Check sheet for the modelled part. Datum: model origin and axes. Units: mm. Face numbers are marked on the shaded views. A direction names the side the tool comes from. Coordinates: 2 decimals unless noted, no trailing zeros. Write each loop counter-clockwise with the first axis right and the second up, starting at its lowest first coordinate (ties: lowest second). Pieces come first, ordered by that corner, then holes. Notation, with made-up numbers: M -32,31.5 L -19,31.5 A13 ccw -19,38.5 Z; hole C 4.25,83.5 d4. An arc over 180 degrees is marked long. Answer as CSV lines item,"result". Start each with the question number.
Q1. Thickness scan on line 1 along X through (y, z) = (7.5, -7.5); line 2 along X through (y, z) = (20, 10.5); line 3 along Y through (x, z) = (-7.25, 10). Record the ranges inside material, lowest first. Write a range as from..to.
Q2. Sectioned sample at A-A, the plane y = 35. Record the cut outline in (x, z), then the cut area to 3 significant figures.
Q3. Access from +Z, -Z, +X, -X, +Y, -Y to the whole of each face (thin tool, end or side, straight path). Record for the marked faces 1, 2, 3 and 4.
Q4. Depth check by flat-ended pin: pin 1 Ø3 at (x, z) = (-5, -7.5) entering from -Y; pin 2 Ø10 at (x, z) = (0, 10) entering from -Y; pin 3 Ø3 at (x, y) = (-1.5, 7.5) entering from +Z; pin 4 Ø0.9 at (x, z) = (3.5, 11.5) entering from -Y. Enter the tip coordinate at first touch or a pass-through.
Q5. Sectioned sample at D-D, the plane x = 5. Record the cut outline in (y, z).
Q6. Sectioned sample at C-C, the plane z = -7.5. Record the cut outline in (x, y), then the cut area to 3 significant figures.
Q7. Sectioned sample at B-B, the plane x = -1.5. Record the cut outline in (y, z), then the cut area to 4 significant figures.
Q8. Mould release check, pull along X, two halves, no side actions. Record for the marked faces 5, 6, 7 and 8: pulls with the +X half, pulls with the -X half, needs draft (parallel to the pull), parting line crosses it, or undercut.
from build123d import *

# Parameters (mm, degrees)
BOSS_EXTRU_1_DEPTH      = 14
ESQUISSE2_W             = 20
ESQUISSE2_H             = 40
BOSS_EXTRU_2_DEPTH      = 15
ENL_V_MAT_EXTRU_1_REACH = 66.384
ENL_V_MAT_EXTRU_2_REACH = 49.418
ESQUISSE4_R             = 2


with BuildPart() as part:
    # Esquisse1 → Boss.-Extru.1 (new body)
    with BuildSketch(Plane(origin=(0, 0, 0), x_dir=(1, 0, 0), z_dir=(0, 1, 0))):
        Polygon((12.5, -12.5), (12.5, 0), (12.5, 12.5), (-12.5, 12.5), (-12.5, -12.5), align=None)
    extrude(amount=BOSS_EXTRU_1_DEPTH)

    # Esquisse2 → Boss.-Extru.2 (add)
    with BuildSketch(Plane.XY.offset(12.5)):
        Polygon((-12.5, 14), (12.5, 14), (12.5, 16.5), (12.5, 58), (-12.5, 58), align=None)
        with Locations((0, 36)):
            Rectangle(ESQUISSE2_W, ESQUISSE2_H, mode=Mode.SUBTRACT)
    extrude(amount=-BOSS_EXTRU_2_DEPTH)

    # Esquisse3 → Enlèv. mat.-Extru.1 (cut, up to next)
    with BuildSketch(Plane.ZY.offset(12.5), mode=Mode.PRIVATE) as enl_v_mat_extru_1_sk1:
        Polygon((12.5, 0), (4.5, 0), (4.5, 10), (9.5, 15), (12.5, 15), align=None)
    enl_v_mat_extru_1_tool1 = extrude(enl_v_mat_extru_1_sk1.sketch, amount=-ENL_V_MAT_EXTRU_1_REACH, mode=Mode.PRIVATE) & part.part
    add(enl_v_mat_extru_1_tool1.solids().sort_by_distance((-12.5, 6.821705, 8.771318))[0], mode=Mode.SUBTRACT)

    # Esquisse4 → Enlèv. mat.-Extru.2 (cut, up to next)
    with BuildSketch(Plane(origin=(0, 14, 0), x_dir=(1, 0, 0), z_dir=(0, 1, 0)), mode=Mode.PRIVATE) as enl_v_mat_extru_2_sk1:
        with Locations(Location((5, 7.5, 0), (0, 0, 270))):
            Circle(ESQUISSE4_R)
    enl_v_mat_extru_2_tool1 = extrude(enl_v_mat_extru_2_sk1.sketch, amount=-ENL_V_MAT_EXTRU_2_REACH, mode=Mode.PRIVATE) & part.part
    # Esquisse4 → Enlèv. mat.-Extru.2 (cut, up to next)
    with BuildSketch(Plane(origin=(0, 14, 0), x_dir=(1, 0, 0), z_dir=(0, 1, 0)), mode=Mode.PRIVATE) as enl_v_mat_extru_2_sk2:
        with Locations(Location((-5, 7.5, 0), (0, 0, 270))):
            Circle(ESQUISSE4_R)
    enl_v_mat_extru_2_tool2 = extrude(enl_v_mat_extru_2_sk2.sketch, amount=-ENL_V_MAT_EXTRU_2_REACH, mode=Mode.PRIVATE) & part.part
    add(enl_v_mat_extru_2_tool1.solids().sort_by_distance((5, 14, -7.5))[0], mode=Mode.SUBTRACT)
    add(enl_v_mat_extru_2_tool2.solids().sort_by_distance((-5, 14, -7.5))[0], mode=Mode.SUBTRACT)


solid = part.part
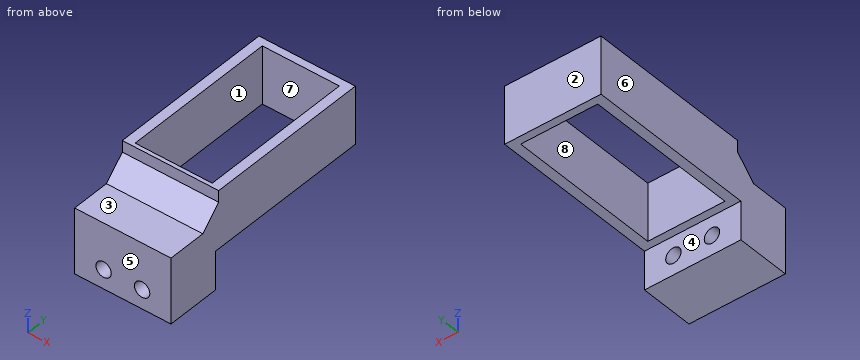
Output:
1,line 1,"x = -12.5..-7, -3..3, 7..12.5"
1,line 2,"x = -12.5..-10, 10..12.5"
1,line 3,"y = 15..16, 56..58"
2,outline,"M -12.5,-2.5 L -10,-2.5 L -10,12.5 L -12.5,12.5 Z; M 10,-2.5 L 12.5,-2.5 L 12.5,12.5 L 10,12.5 Z"
2,area,"75.0 mm^2"
3,face 1,"+Z, -Z"
3,face 2,"+Z, -Z, +X, -X, +Y"
3,face 3,"+Z, +X, -X, -Y"
3,face 4,"-Z, +X, -X, +Y"
4,pin 1,"passes through"
4,pin 2,"stops at y = 10.5"
4,pin 3,"stops at z = 4.5"
4,pin 4,"stops at y = 15"
5,outline,"M 0,-12.5 L 14,-12.5 L 14,-9.5 L 0,-9.5 Z; M 0,-5.5 L 14,-5.5 L 14,-2.5 L 16,-2.5 L 16,12.5 L 15,12.5 L 15,9.5 L 10,4.5 L 0,4.5 Z; M 56,-2.5 L 58,-2.5 L 58,12.5 L 56,12.5 Z"
6,outline,"M -12.5,0 L -7,0 L -7,14 L -12.5,14 Z; M -3,0 L 3,0 L 3,14 L -3,14 Z; M 7,0 L 12.5,0 L 12.5,14 L 7,14 Z"
6,area,"238 mm^2"
7,outline,"M 0,-12.5 L 14,-12.5 L 14,-2.5 L 16,-2.5 L 16,12.5 L 15,12.5 L 15,9.5 L 10,4.5 L 0,4.5 Z; M 56,-2.5 L 58,-2.5 L 58,12.5 L 56,12.5 Z"
7,area,"302.5 mm^2"
8,face 5,"needs draft"
8,face 6,"pulls with the -X half"
8,face 7,"undercut"
8,face 8,"undercut"
